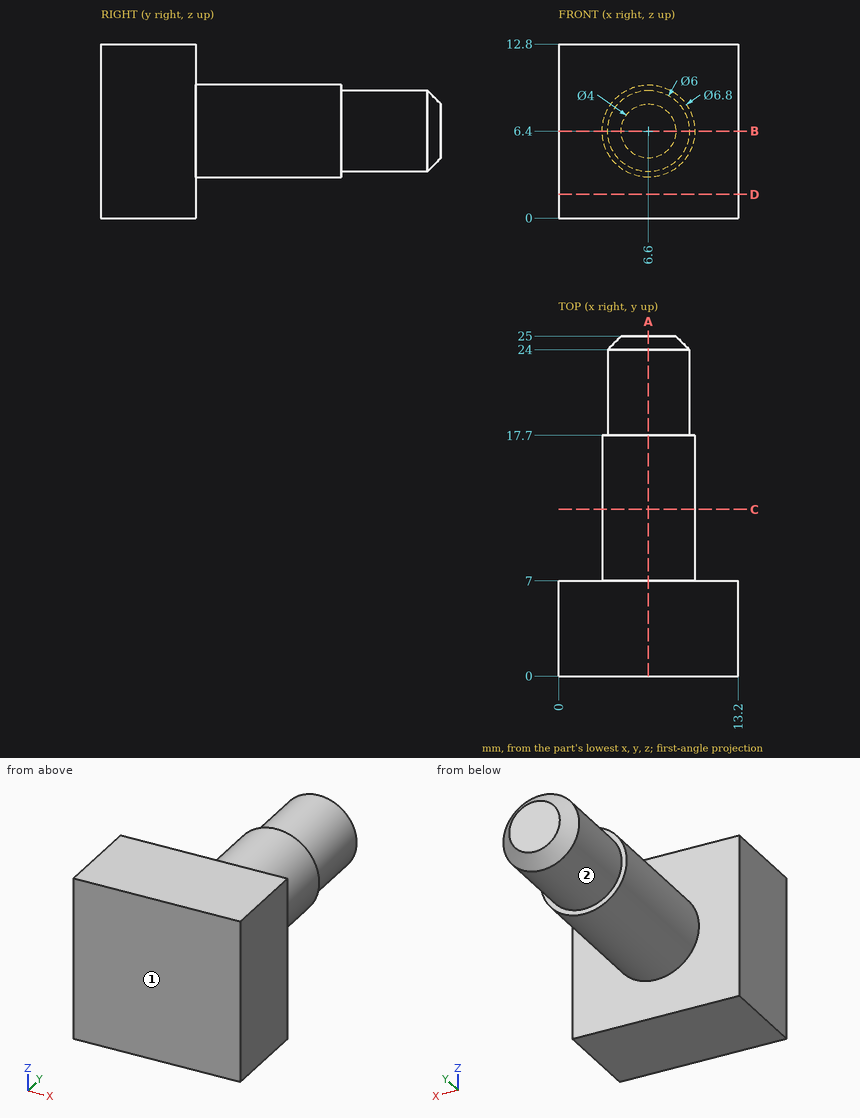
Design review of the part shown in the three views and the two pictorial views. Dimensions are in mm from the part's minimum x, y and z. A direction names the side the tool comes from. Round coordinates to 2 decimals unless told otherwise and drop trailing zeros. Write each loop counter-clockwise with the first axis right and the second up, starting at its lowest first coordinate (ties: lowest second). Pieces come first, ordered by that corner, then holes. Notation, with made-up numbers: (-37, 59) -> (3, 59) arc R22 ccw to (3, 70) -> close; hole circle Ø7 at (-7, 51.25). An arc over 180 degrees is marked (long way). Use one line per item in the form item = value.
1) Tool access review of the marked faces 1 and 2: name each direction out of +Z, -Z, +X, -X, +Y, -Y from which nothing blocks a thin tool from reaching the whole face with its end or side.
Found:
face_1 = +Z, -Z, +X, -X, -Y
face_2 = +Y
2) Take a section at D-D, the plane z = 1.75. Write out the cut boundary in (x, y), and give its area (3 significant figures).
Found:
outline = (0, 0) -> (13.2, 0) -> (13.2, 7) -> (0, 7) -> close
area = 92.4 mm2
3) Clearance check with flat-ended pins moving along their axes: pin 1 (1.5 mm diameter, centred on x = 5.5, y = 13, fed in from -Z); pin 2 (5 mm diameter, centred on y = 16.5, z = 11.5, fed in from -X); pin 3 (6 mm diameter, centred on x = 7.5, z = 2.5, fed in from +Y); pin 4 (3 mm diameter, centred on x = 6, z = 10, fed in from +Y). State where each tip first meets the part, or that it passes through.
Found:
pin_1 = 3.02
pin_2 = 4.41
pin_3 = 25
pin_4 = 24.85
4) Take a section at A-A, the plane x = 6.6. Write out the cut boundary in (y, z), and give its area (3 significant figures).
Found:
outline = (0, 0) -> (7, 0) -> (7, 3) -> (17.7, 3) -> (17.7, 3.4) -> (24, 3.4) -> (25, 4.4) -> (25, 8.4) -> (24, 9.4) -> (17.7, 9.4) -> (17.7, 9.8) -> (7, 9.8) -> (7, 12.8) -> (0, 12.8) -> close
area = 205 mm2
5) To check wall thickness, follow L1, parallel to Y at x = 6.5, z = 1; L2, parallel to X at y = 17.25, z = 5.25; L3, parallel to X at y = 23, z = 5.75. State the ranges of each line that lie inside material, in increasing order. Write a range as from..to.
Found:
L1 = 0..7
L2 = 3.4..9.8
L3 = 3.67..9.53
6) Take a section at C-C, the plane y = 12.25. Write out the cut boundary in (x, z).
Found:
outline = circle Ø6.8 at (6.6, 6.4)
7) Take a section at B-B, the plane z = 6.4. Write out the cut boundary in (x, y), and give its area (3 significant figures).
Found:
outline = (0, 0) -> (13.2, 0) -> (13.2, 7) -> (10, 7) -> (10, 17.7) -> (9.6, 17.7) -> (9.6, 24) -> (8.6, 25) -> (4.6, 25) -> (3.6, 24) -> (3.6, 17.7) -> (3.2, 17.7) -> (3.2, 7) -> (0, 7) -> close
area = 208 mm2
